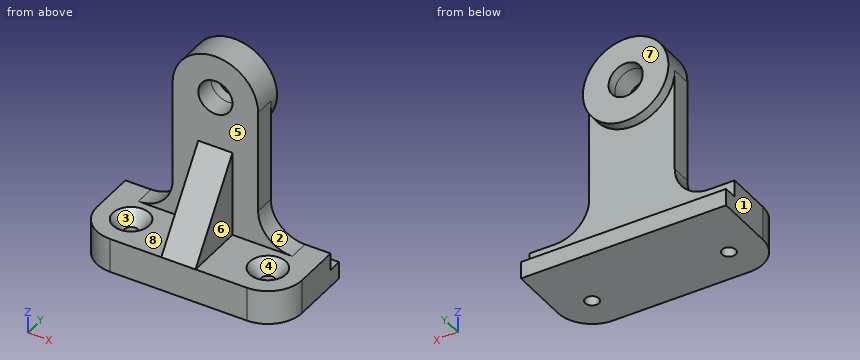
```python
from build123d import *

# Parameters (mm, degrees)
F1_DEPTH        = 29.845
F0_R            = 6.35
F2_DEPTH        = 7.62
F3_W            = 76.2
F3_H            = 6.35
F4_DEPTH        = 5.08
F5_R            = 6.35
F6_DEPTH        = 3.81
F8_DEPTH        = 6.35
F9_R            = 12.7
F11_D           = 5.1054
F11_CSINK_D     = 13.4874
F11_CSINK_ANGLE = 82


with BuildPart() as f1:
    # F0 (on Front) → F1 (new body)
    with BuildSketch(Plane.XZ):
        Polygon((38.1, -50.8), (28.575, -50.8), (-28.575, -50.8), (-38.1, -50.8), (-38.1, -63.5), (38.1, -63.5), align=None)
    extrude(amount=F1_DEPTH)

    # F0 (on Front) → F2 (join)
    with BuildSketch(Plane.XZ):
        with BuildLine():
            Line((15.875, -38.1), (15.875, 0))
            ThreePointArc((15.875, 0), (0, 15.875), (-15.875, 0))
            Line((-15.875, 0), (-15.875, -38.1))
            ThreePointArc((-15.875, -38.1), (-19.5947438789, -47.0802561211), (-28.575, -50.8))
            Line((-28.575, -50.8), (28.575, -50.8))
            ThreePointArc((28.575, -50.8), (19.5947438789, -47.0802561211), (15.875, -38.1))
        make_face()
        Circle(F0_R, mode=Mode.SUBTRACT)
    extrude(amount=F2_DEPTH)

    # F3 (on face) → F4 (join)
    with BuildSketch(Plane(origin=(0, 0, 0), x_dir=(-1, 0, 0), z_dir=(0, 1, 0))):
        with Locations((0, -60.325)):
            Rectangle(F3_W, F3_H)
    extrude(amount=F4_DEPTH)

    # F5 (on face) → F6 (join)
    with BuildSketch(Plane(origin=(0, 0, 0), x_dir=(-1, 0, 0), z_dir=(0, 1, 0))):
        with BuildLine():
            ThreePointArc((15.875, 0), (0, 15.875), (-15.875, 0))
            ThreePointArc((-15.875, 0), (0, -15.875), (15.875, 0))
        make_face()
        Circle(F5_R, mode=Mode.SUBTRACT)
    extrude(amount=F6_DEPTH)

    # F7 (on Right) → F8 (join, symmetric)
    with BuildSketch(Plane.YZ):
        Polygon((-7.62, -50.8), (-7.62, -19.05), (-29.845, -50.8), align=None)
    extrude(amount=F8_DEPTH, both=True)

    # F9
    f9_edges = [f1.edges().sort_by_distance(p)[0] for p in [
        (-38.1, -29.845, -57.15),
        (38.1, -29.845, -57.15),
    ]]
    fillet(f9_edges, radius=F9_R)

    # F11 (through all)
    with Locations(Plane.XY.offset(-50.8)):
        with Locations((25.4, -17.145), (-25.4, -17.145)):
            CounterSinkHole(F11_D / 2, F11_CSINK_D / 2, counter_sink_angle=F11_CSINK_ANGLE)


solid = f1.part
```
The listing builds one solid part. Answer for the finished solid, in the listing's coordinates (mm). Face numbers are marked on the shaded views. A direction names the side the tool comes from. Give positions to 0.01 mm unless a question says otherwise; leave off trailing zeros. Order: outer loops, then holes, each group sorted by start corner. A loop starts at its lowest first (then second) coordinate and runs counter-clockwise, first axis right, second up.
1) For the marked faces 5, 6, 7 and 8, determine the directions among +Z, -Z, +X, -X, +Y, -Y from which every point of the face is accessible in a straight line to the end or side of a thin tool.
Reported:
face 5: +Z, -Y
face 6: +Z, +X, -Y
face 7: +Z, +X, -X, +Y
face 8: +Z, -X, -Y
2) Find section C-C on y = -26. Write down the section's boundary in (x, z).
Reported:
outline: (-34.5, -63.5) - (34.5, -63.5) - (34.5, -50.8) - (6.35, -50.8) - (6.35, -45.31) - (-6.35, -45.31) - (-6.35, -50.8) - (-34.5, -50.8) - close
3) Determine the mould class of the marked faces 1, 2, 3 and 4 for opening direction X: pulls with the +X half, pulls with the -X half, needs draft (parallel to the pull), parting line crosses it, or undercut.
Reported:
face 1: pulls with the -X half
face 2: pulls with the +X half
face 3: undercut
face 4: undercut
4) Consider line 1 along Z through (x, y) = (0, 2.95) (3 decimals); line 2 along Z through (x, y) = (0, -4.5) (3 decimals); line 3 along Z through (x, y) = (14, -28). Determine where each line is inside the solid, lowest interval first.
Reported:
line 1: z = -63.5 to -57.15, -15.875 to -6.35, 6.35 to 15.875
line 2: z = -63.5 to -6.35, 6.35 to 15.875
line 3: z = -63.5 to -50.8
5) Find section D-D on z = -33. Write down the section's boundary in (x, y) (3 decimals).
Reported:
outline: (-15.875, -7.62) - (-6.35, -7.62) - (-6.35, -17.385) - (6.35, -17.385) - (6.35, -7.62) - (15.875, -7.62) - (15.875, 0) - (-15.875, 0) - close
6) Given P1, Ø4, axis at y = -5, z = -11, coming from the +X side (3 decimals); P2, Ø16, axis at x = -5.5, z = -4, coming from the +Y side; P3, Ø1.5, axis at y = -9.5, z = -4, coming from the -X side; P4, Ø8.5, axis at y = -4.5, z = -20, coming from the -X side (3 decimals), each flat-ended and moving along its own axis, determine where each tip first touches the part or whether it passes through.
Reported:
P1: stops at x = 15.875
P2: stops at y = 3.81
P3: passes through
P4: stops at x = -15.875
7) Find section A-A on x = 0. Write down the section's boundary in (y, z) (3 decimals), then the cut area to 3 significant figures.
Reported:
outline: (-29.845, -63.5) - (5.08, -63.5) - (5.08, -57.15) - (0, -57.15) - (0, -15.875) - (3.81, -15.875) - (3.81, -6.35) - (-7.62, -6.35) - (-7.62, -19.05) - (-29.845, -50.8) - close; (-7.62, 6.35) - (3.81, 6.35) - (3.81, 15.875) - (-7.62, 15.875) - close
area: 1,250 mm2
8) Find section B-B on z = 2.5. Write down the section's boundary in (x, y).
Reported:
outline: (-15.68, -7.62) - (-5.84, -7.62) - (-5.84, 3.81) - (-15.68, 3.81) - close; (5.84, -7.62) - (15.68, -7.62) - (15.68, 3.81) - (5.84, 3.81) - close
